Part model, mm, in its own coordinate system. Face numbers are marked on the shaded views. A direction names the side the tool comes from. Give positions to 0.01 mm unless a question says otherwise; leave off trailing zeros. Loops run counter-clockwise (first coordinate to the right, second up) from the corner with the lowest first, then second, coordinate; pieces in that order, holes last. Notation, with made-up numbers: (-38.5, 46.5) -> (3.5, 46.5) arc R16 cw to (3.5, 51.5) -> close; hole circle Ø6 at (-26, 49). An arc over 180 degrees is marked (long way). Write item = value, one per line.
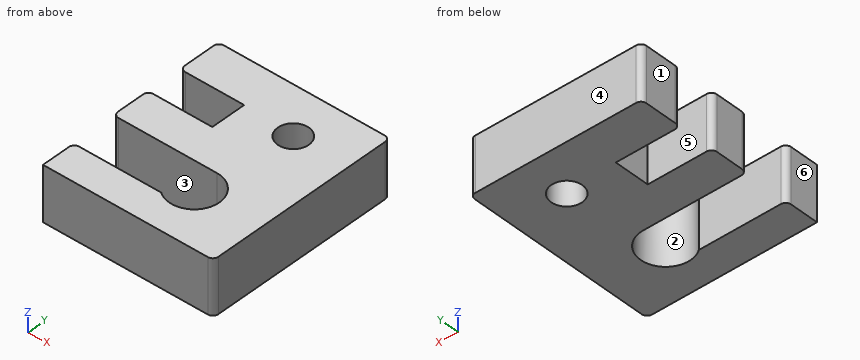
from build123d import *

# Parameters (mm, degrees)
F0_R     = 3.611542
F1_DEPTH = 12.7


with BuildPart() as f1:
    # F0 (on Top) → F1 (new body)
    with BuildSketch(Plane.XY):
        with BuildLine():
            Line((11.588495, 27.25), (-25.871505, 27.25))
            ThreePointArc((-25.871505, 27.25), (-26.769531, 26.878026), (-27.141505, 25.98))
            Line((-27.141505, 25.98), (-27.141505, 18.52))
            ThreePointArc((-27.141505, 18.52), (-26.769531, 17.621974), (-25.871505, 17.25))
            Line((-25.871505, 17.25), (-12.141505, 17.25))
            Line((-12.141505, 17.25), (-12.141505, 9))
            Line((-12.141505, 9), (-25.871505, 9))
            ThreePointArc((-25.871505, 9), (-26.769531, 8.628026), (-27.141505, 7.73))
            Line((-27.141505, 7.73), (-27.141505, 1.27))
            ThreePointArc((-27.141505, 1.27), (-26.769531, 0.371974), (-25.871505, 0))
            Line((-25.871505, 0), (-2.976505, 0))
            ThreePointArc((-2.976505, 0), (2.558271, -7.682559), (-6.481502, -10.5))
            Line((-6.481502, -10.5), (-25.598086, -10.5))
            ThreePointArc((-25.598086, -10.5), (-26.496112, -10.871974), (-26.868086, -11.77))
            Line((-26.868086, -11.77), (-26.868086, -18.462964))
            Line((-26.868086, -18.462964), (11.588495, -18.462964))
            ThreePointArc((11.588495, -18.462964), (12.486521, -18.09099), (12.858495, -17.192964))
            Line((12.858495, -17.192964), (12.858495, 25.98))
            ThreePointArc((12.858495, 25.98), (12.486521, 26.878026), (11.588495, 27.25))
        make_face()
        with Locations((0, 16.488843)):
            Circle(F0_R, mode=Mode.SUBTRACT)
    extrude(amount=F1_DEPTH)


solid = f1.part
1) Which spindle directions (+Z, -Z, +X, -X, +Y, -Y) get a long thin tool onto all of the face, cutting with end or side? Do the marked faces 4, 5 and 6. Say none if no direction does.
Resolved:
face_4 = +Z, -Z, +X, -X, +Y
face_5 = +Z, -Z, -X
face_6 = +Z, -Z, -X, -Y
2) Slice it at D-D, the plane y = -1. List the corners of the cut face in (x, z).
Resolved:
outline = (0.29, 0) -> (12.86, 0) -> (12.86, 12.7) -> (0.29, 12.7) -> close
3) Slice it at B-B, the plane x = -21.5. List the corners of the cut face in (y, z).
Resolved:
outline = (-18.46, 0) -> (-10.5, 0) -> (-10.5, 12.7) -> (-18.46, 12.7) -> close; (0, 0) -> (9, 0) -> (9, 12.7) -> (0, 12.7) -> close; (17.25, 0) -> (27.25, 0) -> (27.25, 12.7) -> (17.25, 12.7) -> close
4) Drill centre lines: line 1 along Y through (x, z) = (-23, 5.5); line 2 along Y through (x, z) = (0, 8.25); line 3 along Y through (x, z) = (-9.5, 3). Where is each one in solid material? Low to high. Write a range as [from, to].
Resolved:
line_1 = [-18.46, -10.5], [0, 9], [17.25, 27.25]
line_2 = [-18.46, -10.85], [-0.82, 12.88], [20.1, 27.25]
line_3 = [-18.46, -10.5], [0, 27.25]
5) Drop flat-ended pins along their axis: P1, Ø2.5, axis at y = 11, z = 6, coming from the -X side; P2, Ø5.5, axis at y = -15.5, z = 9.5, coming from the -X side; P3, Ø4, axis at y = -9.5, z = 9, coming from the -X side. Give the stop position or say it passes through.
Resolved:
P1 = -12.14
P2 = -26.87
P3 = -26.84
6) Slice it at A-A, the plane x = -7. List the corners of the cut face in (y, z), and give its area (3 significant figures).
Resolved:
outline = (-18.46, 0) -> (-10.5, 0) -> (-10.5, 12.7) -> (-18.46, 12.7) -> close; (0, 0) -> (27.25, 0) -> (27.25, 12.7) -> (0, 12.7) -> close
area = 447 mm²
7) Pull direction X, two halves, no side cores. Call the marked faces 1, 2 and 3: pulls with the +X half, pulls with the -X half, needs draft (parallel to the pull), parting line crosses it, or undercut.
Resolved:
face_1 = pulls with the -X half
face_2 = undercut
face_3 = needs draft
